from build123d import *

# Parameters (mm, degrees)
F0_W        = 17.2521322966
F0_H        = 11.3339135423
F1_DEPTH    = 63.5
F2_T1_DEPTH = 116.9691747536
F2_T3_DEPTH = 114.7757874589
F3_SIZE     = 5


# Not quite as in the source:
# - a fillet or chamfer that OpenCascade refuses, or shapes differently, is made with other operations: its cross-section is extruded or revolved along the edge and cut away or added


with BuildPart() as f1:
    # F0 (on Right) → F1 (new body)
    with BuildSketch(Plane.YZ):
        Polygon((-28.8866702467, 39.0534885228), (-43.2048514485, 39.0534885228), (-43.2048514485, 11.3339135423), (-43.2048514485, 0), (16.9898695312, 0), (16.9898695312, 7.7048568055), (8.0409916118, 7.7048568055), (8.0409916118, 19.8725238442), (0.7627514424, 19.8725238442), (0.7627514424, 7.7155772597), (-28.8866702467, 7.7155772597), align=None)
        with Locations((-51.8309175968, 5.6669567712)):
            Rectangle(F0_W, F0_H)
    extrude(amount=F1_DEPTH)

    # F2: fillet of radius 10.8639610307 on 2 edges, made by hand

    # F2_s2 → F2_t1 (cut)
    with BuildSketch(Plane.YZ.offset(-26.7345873768)):
        with BuildLine():
            ThreePointArc((16.9898695312, -2.9889781452), (14.4575061135, 3.9831184184), (8.0409916118, 7.7048568055))
            Line((8.0409916118, 7.7048568055), (16.9898695312, 7.7048568055))
            Line((16.9898695312, 7.7048568055), (16.9898695312, -2.9889781452))
        make_face()
    extrude(amount=F2_T1_DEPTH, mode=Mode.SUBTRACT)

    # F2_s4 → F2_t3 (cut)
    with BuildSketch(Plane.YZ.offset(-25.6378937294)):
        with BuildLine():
            ThreePointArc((8.0409916118, 9.6173663525), (6.0365108418, 15.9050733102), (0.7627514424, 19.8725238442))
            Line((0.7627514424, 19.8725238442), (8.0409916118, 19.8725238442))
            Line((8.0409916118, 19.8725238442), (8.0409916118, 9.6173663525))
        make_face()
    extrude(amount=F2_T3_DEPTH, mode=Mode.SUBTRACT)

    # F3
    f3_edges = [f1.edges().sort_by_distance(p)[0] for p in [
        (31.75, -43.204851, 39.053489),
    ]]
    chamfer(f3_edges, length=F3_SIZE)


solid = f1.part
Could you check a few things on this model? Use its own coordinates, in mm. A direction names the side the tool comes from. Coordinates: 2 decimals unless noted, no trailing zeros. Write each loop counter-clockwise with the first axis right and the second up, starting at its lowest first coordinate (ties: lowest second). Pieces come first, ordered by that corner, then holes. Notation, with made-up numbers: (80, 18) - (122, 18) arc R27 ccw to (122, 55) - close; hole circle Ø9 at (46, 52.5). An arc over 180 degrees is marked (long way). Put each result on its own line as item: value. Start each with the question number.
Q1. I want a section at C-C on y = -10.5. Write out the boundary of the cut face in (x, z), plus the area to 3 significant figures.
Q2. I want a section at A-A on z = 17. Write out the boundary of the cut face in (x, y).
Q3. I want a section at B-B on x = 10. Write out the boundary of the cut face in (y, z).
Q4. I'm going to push flat-ended pins straight in: P1, Ø9.5, axis at x = 19.5, z = 22.5, coming from the +Y side; P2, Ø3.5, axis at x = 28.5, z = 13.5, coming from the -Y side; P3, Ø14, axis at x = 44, y = -48.5, coming from the +Z side. Where does each tip first touch, or does it pass through?
Q5. Thinking about a two-plate mould opening in Y: for faces 4 (the flat face through (31, -28.887, 23)), 5 (the flat face through (31, -60.457, 6)), 6 (the flat face through (31, 8.041, 9)), 7 (the flat face through (0, -31, 11)), which applies, pulls with the +Y half, pulls with the -Y half, needs draft (parallel to the pull), parting line crosses it, or undercut?
Q6. Please list where these lines run through material, in increasing order: L1, parallel to Y at x = 24.5, z = 8.5; L2, parallel to Z at x = 16, y = -19; L3, parallel to Y at x = 23, z = 23.
Q7. I want a section at D-D on z = 22.5. Write out the boundary of the cut face in (x, y), plus the area to 3 significant figures.
Q8. Which directions (+Z, -Z, +X, -X, +Y, -Y) give clear straight access to the entire face, cutting with the end or side of a thin tool? Please do faces 1 (the flat face through (31, -52, 11.334)), 2 (the flat face through (31, -14, 7.716)), 3 (the cylindrical face through (31.305, 13.471, 5.016)).
Checks:
1. outline: (0, 0) - (63.5, 0) - (63.5, 7.72) - (0, 7.72) - close
1. area: 490 mm²
2. outline: (0, -43.2) - (63.5, -43.2) - (63.5, -28.89) - (0, -28.89) - close; (0, 0.76) - (63.5, 0.76) - (63.5, 5.15) - (0, 5.15) - close
3. outline: (-60.46, 0) - (16.57, 0) arc R10.86 ccw to (8.04, 7.7) - (8.04, 9.62) arc R10.86 ccw to (0.76, 19.87) - (0.76, 7.72) - (-28.89, 7.72) - (-28.89, 39.05) - (-38.2, 39.05) - (-43.2, 34.05) - (-43.2, 11.33) - (-60.46, 11.33) - close
4. P1: y = 4.38
4. P2: y = -43.2
4. P3: z = 35.76
5. face 4: undercut
5. face 5: pulls with the -Y half
5. face 6: pulls with the +Y half
5. face 7: needs draft
6. L1: -60.46 to -28.89, 0.76 to 8.04
6. L2: 0 to 7.72
6. L3: -43.2 to -28.89
7. outline: (0, -43.2) - (63.5, -43.2) - (63.5, -28.89) - (0, -28.89) - close
7. area: 909 mm²
8. face 1: +Z, +X, -X, -Y
8. face 2: +Z, +X, -X
8. face 3: +Z, +X, -X, +Y
